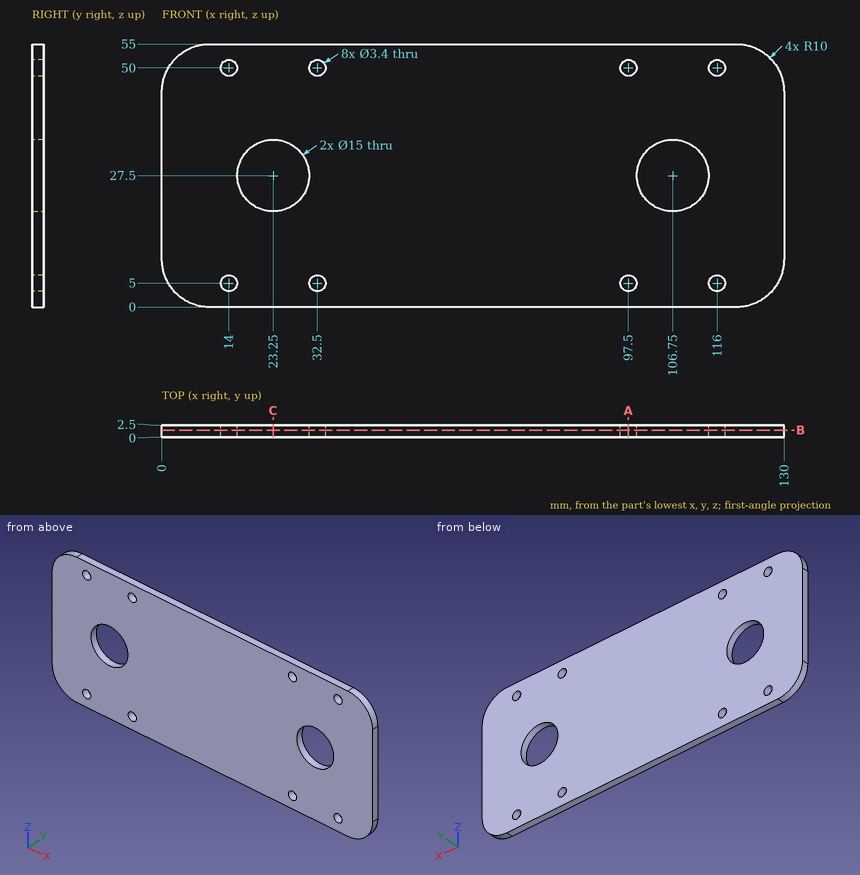
Geometry: see drawing. Coordinates: mm, zero at the bounding-box minimum. Coordinates: 2 decimals unless noted, no trailing zeros. Loops run counter-clockwise (first coordinate to the right, second up) from the corner with the lowest first, then second, coordinate; pieces in that order, holes last.
(1) Section A-A on x = 97.5. Return the cut outline in (y, z).
(2) First-contact query: pin 1 Ø4 at (x, z) = (14, 50) entering from +Y; pin 2 Ø9 at (x, z) = (23.25, 27.5) entering from +Y. Flat tips, straight axial feed; report the tip coordinate or a pass-through.
(3) Section B-B on y = 1.45. Count the separate pieces of the cut face and the enclosed holes in it, then the cut area to 3 significant figures.
(4) Material intervals for probe 1 along X at (y, z) = (1.4, 27.5); probe 2 along Z at (x, y) = (97.5, 1.7); probe 3 along X at (y, z) = (0.85, 50), sorted ascending.
(5) Section C-C on x = 23.25. Return the cut outline in (y, z), then the cut area to 3 significant figures.
Data:
1. outline: (0, 0) - (2.5, 0) - (2.5, 3.3) - (0, 3.3) - close; (0, 6.7) - (2.5, 6.7) - (2.5, 48.3) - (0, 48.3) - close; (0, 51.7) - (2.5, 51.7) - (2.5, 55) - (0, 55) - close
2. pin 1: stops at y = 2.5
2. pin 2: passes through
3. separate pieces: 1
3. enclosed holes: 10
3. area: 6,640 mm2
4. probe 1: x = 0 to 15.75, 30.75 to 99.25, 114.25 to 130
4. probe 2: z = 0 to 3.3, 6.7 to 48.3, 51.7 to 55
4. probe 3: x = 1.34 to 12.3, 15.7 to 30.8, 34.2 to 95.8, 99.2 to 114.3, 117.7 to 128.66
5. outline: (0, 0) - (2.5, 0) - (2.5, 20) - (0, 20) - close; (0, 35) - (2.5, 35) - (2.5, 55) - (0, 55) - close
5. area: 100 mm2
